```python
from build123d import *

# Parameters (mm, degrees)
F0_W     = 5.08
F0_H     = 76.2
F1_DEPTH = 12.7
F2_DEPTH = 5.08
F3_SIZE  = 5.08


with BuildPart() as f1:
    # F0 (on Front) → F1 (new body)
    with BuildSketch(Plane.XZ):
        with Locations((-42.778187, -2.446348)):
            Rectangle(F0_W, F0_H)
    extrude(amount=F1_DEPTH)

    # F0 (on Front) → F2 (join)
    with BuildSketch(Plane.XZ):
        with Locations((-42.778187, -2.446348)):
            Rectangle(F0_W, F0_H)
        Polygon((-52.380648, 43.458667), (-45.318187, 35.653652), (-40.238187, 35.653652), (-33.673275, 43.458667), (-40.238187, 69.648996), (-45.318187, 69.648996), align=None)
    extrude(amount=F2_DEPTH)

    # F3
    f3_edges = [f1.edges().sort_by_distance(p)[0] for p in [
        (-42.778187, -12.7, 35.653652),
    ]]
    chamfer(f3_edges, length=F3_SIZE)


solid = f1.part
```
For this review, take the finished solid that the model builds, in its own axes (mm). A direction names the side the tool comes from. Give positions to 0.01 mm unless a question says otherwise; leave off trailing zeros. Write each loop counter-clockwise with the first axis right and the second up, starting at its lowest first coordinate (ties: lowest second). Pieces come first, ordered by that corner, then holes. Notation, with made-up numbers: M -23.75,57.25 L 32.25,57.25 A15 cw 32.25,77.25 Z; hole C 55,44.25 d3. An arc over 180 degrees is marked long. One line per item, written item: value.
1) For P1, Ø1.5, axis at y = -5, z = -15, coming from the -X side; P2, Ø6.5, axis at y = -4.5, z = 4, coming from the +X side, all flat-tipped, find the tip position at first contact; note any pin that passes through.
Results are:
P1: stops at x = -45.32
P2: stops at x = -40.24
2) Take a section at C-C, the plane z = 47. Write out the cut boundary in (x, y).
Results are:
outline: M -51.43,-5.08 L -34.56,-5.08 L -34.56,0 L -51.43,0 Z
3) For faces 1 (the flat face through (-43, -5.08, 53)), 2 (the flat face through (-43, -12.7, -4)), 3 (the flat face through (-45.318, -6, -3)), 4 (the flat face through (-40.238, -6, -3)), list the 3-axis set-ups (+Z, -Z, +X, -X, +Y, -Y) from which the entire face can be reached by the end or side of a thin tool; tool diameter is ignored.
Results are:
face 1: +Z, +X, -X, -Y
face 2: +Z, -Z, +X, -X, -Y
face 3: -Z, -X, +Y, -Y
face 4: -Z, +X, +Y, -Y
4) Take a section at B-B, the plane x = -42. Write out the cut boundary in (y, z), then the cut area to 3 significant figures.
Results are:
outline: M -12.7,-40.55 L 0,-40.55 L 0,69.65 L -5.08,69.65 L -5.08,35.65 L -7.62,35.65 L -12.7,30.57 Z
area: 1,130 mm²
5) Take a section at A-A, the plane y = -1.25. Write out the cut boundary in (x, z), then the cut area to 3 significant figures.
Results are:
outline: M -52.38,43.46 L -45.32,35.65 L -45.32,-40.55 L -40.24,-40.55 L -40.24,35.65 L -33.67,43.46 L -40.24,69.65 L -45.32,69.65 Z
area: 791 mm²
6) Take a section at D-D, the plane y = -6. Write out the cut boundary in (x, z), then the cut area to 3 significant figures.
Results are:
outline: M -45.32,-40.55 L -40.24,-40.55 L -40.24,35.65 L -45.32,35.65 Z
area: 387 mm²
7) For line 1 (X direction, y = -9.5, z = -5); line 2 (Y direction, x = -45.75, z = 64); line 3 (Z direction, x = -43.5, y = -9.75), list the stretches that pass through material, from the lowest coordinate up. Write a range as from..to.
Results are:
line 1: x = -45.32..-40.24
line 2: y = -5.08..0
line 3: z = -40.55..33.52
